```python
from build123d import *

# Parameters (mm, degrees)
F1_DEPTH = 15
F2_R     = 8
F3_DEPTH = 240
F4_SIZE  = 2


with BuildPart() as f1:
    # F0 (on Front) → F1 (new body)
    with BuildSketch(Plane.XZ):
        Polygon((-15.588133, 0.100479), (-7.881084, -13.44948), (7.707049, -13.549959), (15.588133, -0.100479), (7.881084, 13.44948), (-7.707049, 13.549959), align=None)
    extrude(amount=-F1_DEPTH)

    # F2 (on face) → F3 (join)
    with BuildSketch(Plane.XZ):
        Circle(F2_R)
    extrude(amount=F3_DEPTH)

    # F4
    f4_edges = [f1.edges().sort_by_distance(p)[0] for p in [
        (-8, -240, 0),
    ]]
    chamfer(f4_edges, length=F4_SIZE)


solid = f1.part
```
Model file for the job. Use its own axes, mm. A direction names the side the tool comes from. Coordinates: 2 decimals unless noted, no trailing zeros. Order: outer loops, then holes, each group sorted by start corner. A loop starts at its lowest first (then second) coordinate and runs counter-clockwise, first axis right, second up. Notation, with made-up numbers: (14.5, 55) -> (28.5, 55) arc R21 cw to (28.5, 90) -> close; hole circle Ø10 at (-4.75, 58). An arc over 180 degrees is marked (long way). Answer as a JSON object with one key per item and string values. Group by question number.
1) Flat gauge pins, fed straight in: pin 1 (6 mm diameter, centred on y = -182, z = 10, fed in from -X); pin 2 (1.5 mm diameter, centred on x = -7, z = -10.5, fed in from -Y); pin 3 (12 mm diameter, centred on y = -133, z = 4.5, fed in from +X). Where does each tip first touch, or does it go through?
2) Which spindle directions (+Z, -Z, +X, -X, +Y, -Y) get a long thin tool onto all of the face, cutting with end or side? Do faces 1 (the face through (-11.59, 7.4, 6.92)), 2 (the face through (-1.73, -117.33, -7.81)). Say none if no direction does.
3) Drill centre lines: L1, parallel to Y at x = -7, z = 9.5; L2, parallel to Z at x = 0, y = -47; L3, parallel to Y at x = 3, z = 5.25. Where is each one in solid material? Low to high.
4) Cut at A-A, the plane y = -134. Write the cut outline in (x, z), then the cut area to 3 significant figures.
5) Cut at C-C, the plane x = 12.5. Write the cut outline in (y, z), then the cut area to 3 significant figures.
6) Cut at B-B, the plane x = 0. Write the cut outline in (y, z).
Check values:
{
 "1": {"pin 1": "stops at x = -3.87", "pin 2": "stops at y = 0", "pin 3": "stops at x = 8"},
 "2": {"face 1": "+Z, -X, +Y, -Y", "face 2": "-Y"},
 "3": {"L1": "y = 0 to 15", "L2": "z = -8 to 8", "L3": "y = -239.95 to 15"},
 "4": {"outline": "circle Ø16 at (0, 0)", "area": "201 mm²"},
 "5": {"outline": "(0, -5.37) -> (15, -5.37) -> (15, 5.33) -> (0, 5.33) -> close", "area": "160 mm²"},
 "6": {"outline": "(-240, -6) -> (-238, -8) -> (0, -8) -> (0, -13.5) -> (15, -13.5) -> (15, 13.5) -> (0, 13.5) -> (0, 8) -> (-238, 8) -> (-240, 6) -> close"}
}
